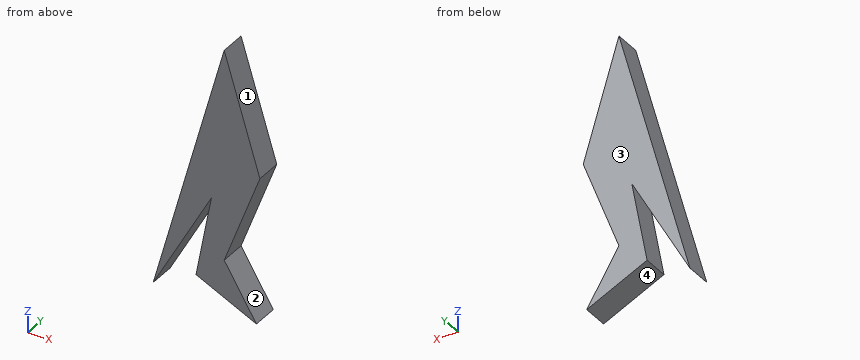
from build123d import *

# Parameters (mm, degrees)
F2_DEPTH = 25.4


with BuildPart() as f2:
    # F1 (on face) → F2 (new body)
    with BuildSketch(Plane.XZ):
        with BuildLine():
            Line((33.595659, -109.857202), (0, 0))
            Line((0, 0), (-66.741718, -241.01392))
            ThreePointArc((-66.741718, -241.01392), (-66.715884, -241.021072), (-66.69005, -241.028222))
            Line((-66.69005, -241.028222), (-12.01611, -143.133894))
            Line((-12.01611, -143.133894), (-26.489001, -220.296562))
            Line((-26.489001, -220.296562), (30.318644, -247.961536))
            Line((30.318644, -247.961536), (0, -197.876692))
            Line((0, -197.876692), (33.595659, -109.857202))
        make_face()
    extrude(amount=F2_DEPTH)


solid = f2.part
Geometry: final body of the model. Coordinates: model frame, mm. Face numbers are marked on the shaded views. Give positions to 0.01 mm unless a question says otherwise; leave off trailing zeros. Loops run counter-clockwise (first coordinate to the right, second up) from the corner with the lowest first, then second, coordinate; pieces in that order, holes last. Notation, with made-up numbers: (34.25, -25) - (70.25, -25) arc R24 cw to (70.25, 5) - close; hole circle Ø5 at (89, 72). An arc over 180 degrees is marked (long way). One line per question, with ' | ' between items. Start each with the question number.
(1) Section query C-C on y = -16.5. Return loops of the section in (x, z), then the cut area to 3 significant figures.
(2) Section query A-A on z = -150. Return loops of the section in (x, y).
(3) Pull-direction query (Z, two-part tool) for the marked faces 1, 2, 3 and 4; classes: released by +Z, released by -Z, zero draft, split by the parting line, or undercut.
(4) Section query B-B on x = 8. Return loops of the section in (y, z).
(5) Ray query, line 1 (X direction, y = -12.25, z = -158.5); line 2 (X direction, y = -3.25, z = -206.5); line 3 (X direction, y = -8.5, z = -86). Return the intervals inside material, ascending. Write a range as from..to.
(6) Section query D-D on x = -52.5. Return loops of the section in (y, z), then the cut area to 3 significant figures.
(7) Contact query for flat-ended pins moving along their axis: pin 1 (6 mm diameter, centred on y = -10.5, z = -38, fed in from +X); pin 2 (5 mm diameter, centred on x = -27.5, y = -12, fed in from -Z); pin 3 (6 mm diameter, centred on y = -3, z = -175.5, fed in from +X); pin 4 (1.5 mm diameter, centred on x = 3.5, z = -206.5, fed in from +Y). Output: stop coordinate, or through.
The answers:
1) outline: (-66.74, -241.01) arc R372.78 ccw to (-66.69, -241.03) - (-12.02, -143.13) - (-26.49, -220.3) - (30.32, -247.96) - (0, -197.88) - (33.6, -109.86) - (0, 0) - close | area: 9,710 mm2
2) outline: (-41.54, -25.4) - (-15.85, -25.4) - (-15.85, 0) - (-41.54, 0) - close; (-13.3, -25.4) - (18.27, -25.4) - (18.27, 0) - (-13.3, 0) - close
3) face 1: released by +Z | face 2: undercut | face 3: zero draft | face 4: released by -Z
4) outline: (-25.4, -237.09) - (0, -237.09) - (0, -211.09) - (-25.4, -211.09) - close; (-25.4, -176.92) - (0, -176.92) - (0, -26.16) - (-25.4, -26.16) - close
5) line 1: -43.89..-20.6, -14.9..15.03 | line 2: -57.18..-47.41, -23.9..5.22 | line 3: -23.82..26.3
6) outline: (-25.4, -215.62) - (0, -215.62) - (0, -189.59) - (-25.4, -189.59) - close | area: 661 mm2
7) pin 1: x = 12.54 | pin 2: z = -221.02 | pin 3: x = 9.69 | pin 4: y = 0
